Work out the finished part from the listing and answer in its coordinate system (mm). A direction names the side the tool comes from. Coordinates: 2 decimals unless noted, no trailing zeros. Loops run counter-clockwise (first coordinate to the right, second up) from the corner with the lowest first, then second, coordinate; pieces in that order, holes last. Notation, with made-up numbers: (32.25, 6.5) - (80.25, 6.5) arc R17 cw to (80.25, 13.5) - close; hole circle Ø9 at (14.25, 38). An arc over 180 degrees is marked (long way). Write each question's results on one line, items separated by ' | '. Start each with the question number.
1. This flat-tipped pin is pushed along its axis until it touches: P1, Ø8, axis at y = 32, z = -23.5, coming from the +X side. Where does it stop, or does it pass through?
2. Determine the mould class of faces 1 (the flat face through (1, -1, 42.5)), 2 (the flat face through (-1, -1, -39.5)), 3 (the flat face through (1, -67.5, -1)), 4 (the flat face through (-1, -1, 39.5)) for opening direction Y: released by +Y, released by -Y, zero draft, split by the parting line, or undercut.
3. A cutting plane is placed at C-C on z = 18. State how many separate pieces and enclosed holes the cut face has, then the cut area to 3 significant figures.
4. Which of the six approach directions +Z, -Z, +X, -X, +Y, -Y give full straight-line access (tool end or side, diameter ignored) to faces 5 (the flat face through (1, -1, -42.5)), 6 (the flat face through (12, 66, -1))?
5. Find the intervals of material crossed by line 1 along Y through (x, z) = (9.5, 7.5); line 2 along Z through (x, y) = (-0.25, -24.5); line 3 along Z through (x, y) = (13.25, 21), in increasing order. Write a range as [from, to].
6. A cutting plane is placed at A-A on x = -5.75. Determine the outline of the cut face in (y, z), then the cut area to 3 significant figures.
7. A cutting plane is placed at B-B on y = -47. Determine the outline of the cut face in (x, z).
from build123d import *

# Parameters (mm, degrees)
F0_W     = 135
F0_H     = 85
F1_DEPTH = 14
F2_W     = 129
F2_H     = 79
F3_DEPTH = 26
F4_W     = 132
F4_H     = 82
F4_W_2   = 129
F4_H_2   = 79
F5_DEPTH = 3
F6_W     = 4
F6_H     = 71
F7_DEPTH = 25
F8_DEPTH = 1
F9_DEPTH = 1


with BuildPart() as f1:
    # F0 (on Right) → F1 (new body, symmetric)
    with BuildSketch(Plane.YZ):
        Rectangle(F0_W, F0_H)
    extrude(amount=F1_DEPTH, both=True)

    # F2 (on face) → F3 (cut)
    with BuildSketch(Plane.YZ.offset(14)):
        Rectangle(F2_W, F2_H)
    extrude(amount=-F3_DEPTH, mode=Mode.SUBTRACT)

    # F4 (on face) → F5 (cut)
    with BuildSketch(Plane.YZ.offset(14)):
        Rectangle(F4_W, F4_H)
        Rectangle(F4_W_2, F4_H_2, mode=Mode.SUBTRACT)
    extrude(amount=-F5_DEPTH, mode=Mode.SUBTRACT)

    # F6 (on face) → F7 (cut)
    with BuildSketch(Plane(origin=(-14, 0, 0), x_dir=(0, -1, 0), z_dir=(-1, 0, 0))):
        with Locations((-58.5, 0)):
            Rectangle(F6_W, F6_H)
        with Locations((-51, 0)):
            Rectangle(F6_W, F6_H)
        with Locations((-43.5, 0)):
            Rectangle(F6_W, F6_H)
        with Locations((-36, 0)):
            Rectangle(F6_W, F6_H)
        with Locations((-28.5, 0)):
            Rectangle(F6_W, F6_H)
        with Locations((-21, 0)):
            Rectangle(F6_W, F6_H)
        with Locations((-13.5, 0)):
            Rectangle(F6_W, F6_H)
        with Locations((-6, 0)):
            Rectangle(F6_W, F6_H)
        with Locations((43.5, 0)):
            Rectangle(F6_W, F6_H)
        with Locations((21, 0)):
            Rectangle(F6_W, F6_H)
        with Locations((28.5, 0)):
            Rectangle(F6_W, F6_H)
        with Locations((13.5, 0)):
            Rectangle(F6_W, F6_H)
        with Locations((58.5, 0)):
            Rectangle(F6_W, F6_H)
        with Locations((36, 0)):
            Rectangle(F6_W, F6_H)
        with Locations((51, 0)):
            Rectangle(F6_W, F6_H)
        with Locations((6, 0)):
            Rectangle(F6_W, F6_H)
    extrude(amount=-F7_DEPTH, mode=Mode.SUBTRACT)

    # F8 (cut): a face of the model
    f8_faces = [f1.faces().sort_by_distance(p)[0] for p in [
        (-14, 0, 0),
    ]]
    extrude(f8_faces, amount=-F8_DEPTH, mode=Mode.SUBTRACT)

    # F9 (cut): a face of the model
    f9_faces = [f1.faces().sort_by_distance(p)[0] for p in [
        (11, 0, 40.8446037323),
    ]]
    extrude(f9_faces, amount=-F9_DEPTH, mode=Mode.SUBTRACT)


solid = f1.part
Values:
1) P1: x = -12
2) face 1: zero draft | face 2: undercut | face 3: released by -Y | face 4: undercut
3) separate pieces: 17 | enclosed holes: 0 | area: 215 mm^2
4) face 5: -Z, +X, -X, +Y, -Y | face 6: +X
5) line 1: [-67.5, -64.5], [64.5, 67.5] | line 2: [-42.5, -39.5], [39.5, 42.5] | line 3: [-42.5, -41], [41, 42.5]
6) outline: (-67.5, -42.5) - (67.5, -42.5) - (67.5, 42.5) - (-67.5, 42.5) - close; hole (-64.5, -39.5) - (64.5, -39.5) - (64.5, 39.5) - (-64.5, 39.5) - close | area: 1,280 mm^2
7) outline: (-13, -42.5) - (14, -42.5) - (14, -41) - (10, -41) - (10, -39.5) - (-12, -39.5) - (-12, 39.5) - (10, 39.5) - (10, 41) - (14, 41) - (14, 42.5) - (-13, 42.5) - close
